Part print with two shaded views. Sizes in mm from the minimum x, y, z corner. A direction names the side the tool comes from. Give positions to 0.01 mm unless a question says otherwise; leave off trailing zeros. Write each loop counter-clockwise with the first axis right and the second up, starting at its lowest first coordinate (ties: lowest second). Pieces come first, ordered by that corner, then holes.
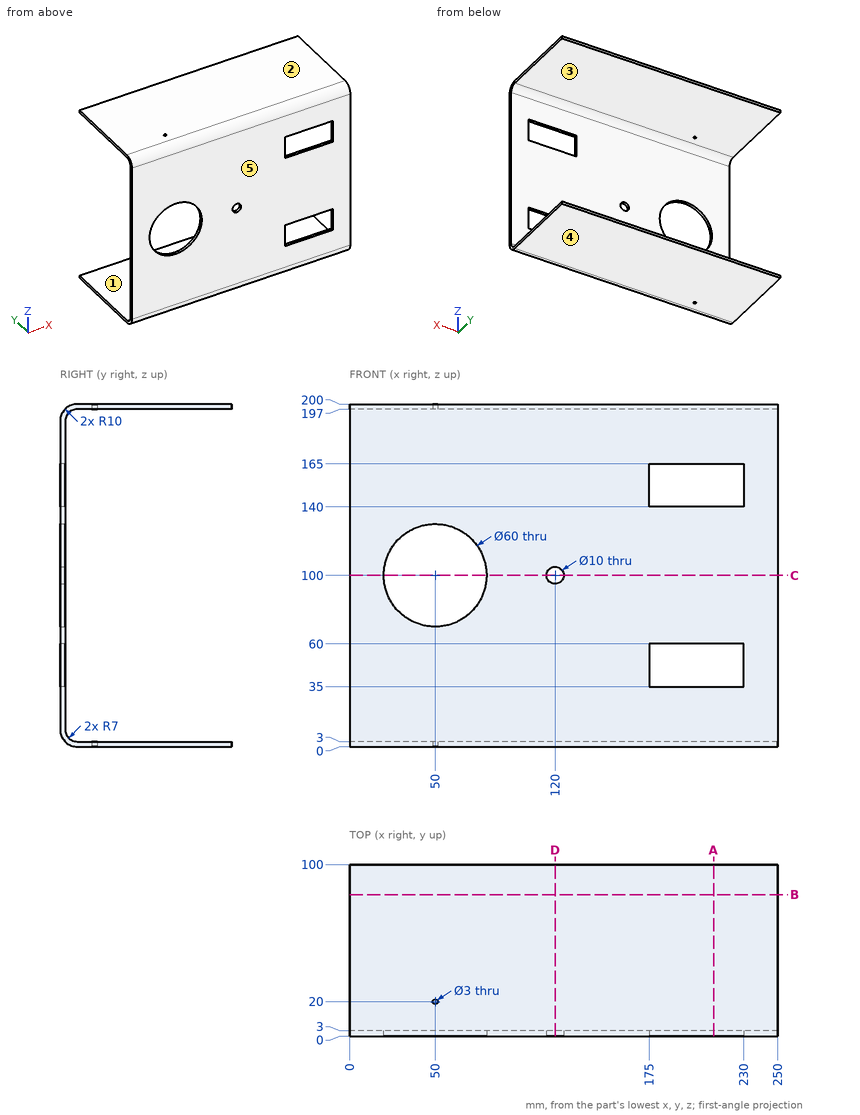
1) Saw through at C-C, the plane z = 100. Write the cut outline in (x, y).
Answers follow:
outline: (0, 0) - (20, 0) - (20, 3) - (0, 3) - close; (80, 0) - (115, 0) - (115, 3) - (80, 3) - close; (125, 0) - (250, 0) - (250, 3) - (125, 3) - close
2) Saw through at D-D, the plane x = 120. Write the cut outline in (y, z).
Answers follow:
outline: (0, 10) arc R10 ccw to (10, 0) - (100, 0) - (100, 3) - (10, 3) arc R7 cw to (3, 10) - (3, 95) - (0, 95) - close; (0, 105) - (3, 105) - (3, 190) arc R7 cw to (10, 197) - (100, 197) - (100, 200) - (10, 200) arc R10 ccw to (0, 190) - close
3) Pin check, flat tips, straight feed: pin 1 Ø3.5 at (x, y) = (216, 1.5) entering from +Z; pin 2 Ø0.9 at (x, y) = (212, 2) entering from +Z; pin 3 Ø1 at (x, z) = (218.5, 126.5) entering from +Y. Stop position of each tip, or through.
Answers follow:
pin 1: stops at z = 197.38
pin 2: stops at z = 196.56
pin 3: stops at y = 3
4) Wall check: L1, parallel to X at y = 1, z = 100; L2, parallel to Z at x = 59.5, y = 71; L3, parallel to X at y = 20, z = 1.55. Give the ranges that are in metal, low to high.
Answers follow:
L1: x = 0 to 20, 80 to 115, 125 to 250
L2: z = 0 to 3, 197 to 200
L3: x = 0 to 48.5, 51.5 to 250
5) Two-plate mould, pull along Z, no slides. Class the marked faces 3, 4 and 5: +Z half, -Z half, draft (parallel to the pull), parting line (faces both ways), or undercut.
Answers follow:
face 3: undercut
face 4: -Z half
face 5: draft
6) Saw through at B-B, the plane y = 82.5. Write the cut outline in (x, z), then the cut area to 3 significant figures.
Answers follow:
outline: (0, 0) - (250, 0) - (250, 3) - (0, 3) - close; (0, 197) - (250, 197) - (250, 200) - (0, 200) - close
area: 1,500 mm2
7) 3-axis set-ups, long thin cutter, end or side, ignore diameter. For the marked faces 1 and 2: which of +Z, -Z, +X, -X, +Y, -Y reach the whole face in a straight line?
Answers follow:
face 1: +X, -X, +Y
face 2: +Z, +X, -X, +Y, -Y
8) Saw through at A-A, the plane x = 212.5. Write the cut outline in (y, z).
Answers follow:
outline: (0, 10) arc R10 ccw to (10, 0) - (100, 0) - (100, 3) - (10, 3) arc R7 cw to (3, 10) - (3, 35) - (0, 35) - close; (0, 60) - (3, 60) - (3, 140) - (0, 140) - close; (0, 165) - (3, 165) - (3, 190) arc R7 cw to (10, 197) - (100, 197) - (100, 200) - (10, 200) arc R10 ccw to (0, 190) - close
